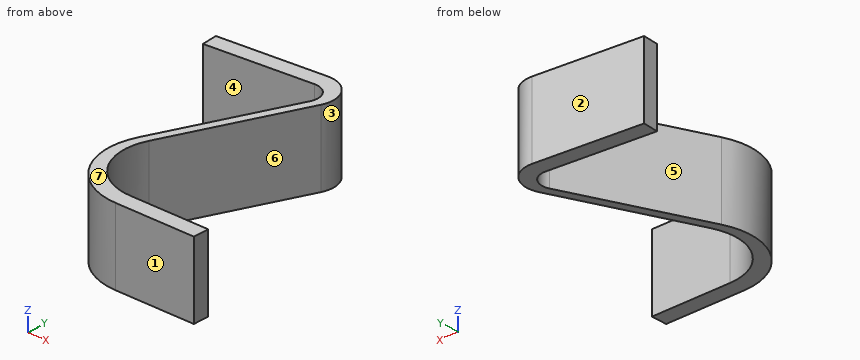
```python
from build123d import *

# Parameters (mm, degrees)
BOSS_EXTRUDE1_DEPTH      = 7
BOSS_EXTRUDE1_DEPTH_BACK = 7


with BuildPart() as part:
    # Sketch1 → Boss-Extrude1 (new, two sides: drawn at the far end of the back side and taken through both)
    with BuildSketch(Plane.XY.offset(-BOSS_EXTRUDE1_DEPTH_BACK)):
        with BuildLine():
            Line((-17.458418155, -11.36484808), (2.465475807, -9.621733225))
            ThreePointArc((2.465475807, -9.621733225), (6.955793602, -11.676837129), (7.491085956, -16.585998774))
            Line((7.491085956, -16.585998774), (-3.072780906, -41.033415882))
            ThreePointArc((-3.072780906, -41.033415882), (-2.24972743, -50.492456592), (6.106881965, -55))
            Line((6.106881965, -55), (21.106881965, -55))
            Line((21.106881965, -55), (21.106881965, -58))
            Line((21.106881965, -58), (6.106881965, -58))
            ThreePointArc((6.106881965, -58), (-3.921049309, -52.59094791), (-4.908713481, -41.240099059))
            Line((-4.908713481, -41.240099059), (5.655153382, -16.79268195))
            ThreePointArc((5.655153382, -16.79268195), (5.333977969, -13.847184963), (2.639787292, -12.614122621))
            Line((2.639787292, -12.614122621), (-17.197282581, -14.349641352))
            Line((-17.197282581, -14.349641352), (-17.458418155, -11.36484808))
        make_face()
    extrude(amount=BOSS_EXTRUDE1_DEPTH + BOSS_EXTRUDE1_DEPTH_BACK)


solid = part.part
```
For this review, take the finished solid that the model builds, in its own axes (mm). Face numbers are marked on the shaded views. A direction names the side the tool comes from. Give positions to 0.01 mm unless a question says otherwise; leave off trailing zeros. Write each loop counter-clockwise with the first axis right and the second up, starting at its lowest first coordinate (ties: lowest second). Pieces come first, ordered by that corner, then holes.
Item 1: Machinability: for the marked faces 4, 5, 6 and 7, which of the approach directions +Z, -Z, +X, -X, +Y, -Y give a long, thin tool a straight path to every point of the face, cutting with its end or side? Answer none if there is none.
Item 2: Take a section at D-D (y = -50.5). Give the boundary of the cut face in (x, z).
Item 3: Take a section at B-B (z = -0.5). Give the boundary of the cut face in (x, y).
Item 4: The part is to be moulded in two halves that separate along Y. For the marked faces 1, 2 and 3, say which applies: +Y half, -Y half, draft (parallel to the pull), parting line (faces both ways), or undercut.
Item 5: Insertion check: P1, Ø1, axis at x = -3, z = -4.5, coming from the -Y side; P2, Ø6, axis at y = -47.5, z = 0.5, coming from the +X side; P3, Ø4, axis at x = 12.5, z = 0.5, coming from the +Y side; P4, Ø10, axis at x = 3, y = -41.5, coming from the +Z side. Each pin has a flat end and moves straight along its axis. Give the tip position at first contact, or say it passes through.
Item 6: Take a section at C-C (x = 12). Give the boundary of the cut face in (y, z).
Item 7: Take a section at A-A (x = 3.5). Give the boundary of the cut face in (y, z).
Item 8: Wall thickness on probe 1 along Y at (x, z) = (2.5, -1.75); probe 2 along Y at (x, z) = (6, 2.75); probe 3 along Y at (x, z) = (18, 2.25): over which ranges is each line inside the solid? List them lowest first.
Established:
1. face 4: +Z, -Z
1. face 5: +Z, -Z, -X
1. face 6: +Z, -Z, +X
1. face 7: +Z, +X, -X, +Y, -Y
2. outline: (-5.02, -7) - (-2.24, -7) - (-2.24, 7) - (-5.02, 7) - close
3. outline: (-17.46, -11.36) - (-17.2, -14.35) - (2.64, -12.61) arc R3 cw to (5.66, -16.79) - (-4.91, -41.24) arc R12 ccw to (6.11, -58) - (21.11, -58) - (21.11, -55) - (6.11, -55) arc R10 cw to (-3.07, -41.03) - (7.49, -16.59) arc R5 ccw to (2.47, -9.62) - close
4. face 1: -Y half
4. face 2: +Y half
4. face 3: undercut
5. P1: stops at y = -54.36
5. P2: stops at x = -2.24
5. P3: stops at y = -55
5. P4: passes through
6. outline: (-58, -7) - (-55, -7) - (-55, 7) - (-58, 7) - close
7. outline: (-57.71, -7) - (-54.65, -7) - (-54.65, 7) - (-57.71, 7) - close; (-25.82, -7) - (-21.78, -7) - (-21.78, 7) - (-25.82, 7) - close; (-12.66, -7) - (-9.64, -7) - (-9.64, 7) - (-12.66, 7) - close
8. probe 1: y = -57.45 to -54.33, -28.14 to -24.09, -12.63 to -9.62
8. probe 2: y = -58 to -55, -20.04 to -10.68
8. probe 3: y = -58 to -55
